Autodesk Inventor part; units mm, degrees
ref_plane "YZ Plane" through (0, 0, 0) normal (1, 0, 0) x (0, 1, 0)
ref_plane "XZ Plane" through (0, 0, 0) normal (0, 1, 0) x (-1, 0, 0)
ref_plane "XY Plane" through (0, 0, 0) normal (0, 0, 1) x (1, 0, 0)
sketch "Sketch1" plane through (0, 0, 0) normal (0, 1, 0) x (-1, 0, 0)
  line L0 (-31, -18.5) -> (31, -18.5)
  line L1 (31, -18.5) -> (31, 18.5)
  line L2 (31, 18.5) -> (-31, 18.5)
  line L3 (-31, 18.5) -> (-31, -18.5)
  line L4 (-31, -18.5) -> (31, 18.5) construction
  line L5 (31, -18.5) -> (-31, 18.5) construction
  line L6 (-35, -22) -> (35, -22)
  line L7 (35, -22) -> (35, 22)
  line L8 (35, 22) -> (-35, 22)
  line L9 (-35, 22) -> (-35, -22)
  line L10 (-35, -22) -> (35, 22) construction
  line L11 (35, -22) -> (-35, 22) construction
  line L12 (12.5, -32) -> (-12.5, -32)
  line L13 (0, -22) -> (12.5, -32) construction
  line L14 (0, -22) -> (-12.5, -32) construction
  line L15 (-12.5, 32) -> (12.5, 32)
  line L16 (12.5, 32) -> (12.5, 22)
  line L17 (-12.5, 22) -> (-12.5, 32)
  line L18 (-12.5, 32) -> (0, 22) construction
  line L19 (12.5, 32) -> (0, 22) construction
  line L20 (12.5, -22) -> (12.5, -32)
  line L21 (-12.5, -32) -> (-12.5, -22)
  line L22 (-12.5, -27) -> (12.5, -27)
  line L23 (-12.5, 27) -> (12.5, 27)
  line L24 (-35, -22) -> (-35, -18.5)
  line L25 (-35, 22) -> (-31, 22)
  line L26 (-35, 22) -> (-35, 18.5)
  point P0 (0, 0)
  dimension "d2" = 70
  dimension "d3" = 44
  dimension "d16" = 25
  dimension "d97" = 37
extrude "Extrusion2" add sketch "Sketch1" along normal blind 20 contours L9 L8 L7 L6
extrude "Extrusion3" add sketch "Sketch1" along normal blind 2 contours L3 L2 L1 L0
sketch "Sketch2" plane through (-35, 0, 22) normal (0, 0, 1) x (1, 0, 0)
  line L0 (66, 2) -> (66, 20)
  line L1 (4, 2) -> (4, 20)
  line L2 (66, 13.7796) -> (4, 13.7796)
  line L3 (4, 13.7796) -> (4, 6.7329)
  line L4 (4, 6.7329) -> (66, 6.7329)
  line L5 (66, 6.7329) -> (66, 13.7796)
  point P0 (35, 0)
extrude "Extrusion4" cut sketch "Sketch2" against normal blind 45
extrude "Extrusion5" add sketch "Sketch1" along normal blind 2 contours L6 L20 L22 L21 | L22 L20 L12 L21
extrude "Extrusion6" add sketch "Sketch1" along normal blind 2 contours L8 L17 L23 L16 | L23 L17 L15 L16
sketch "Sketch3" plane through (-12.5, 2, 32) normal (0, 0, 1) x (1, 0, 0)
  line L0 (2.5, -3.3793) -> (22.5, -3.3793)
  line L1 (22.5, -3.3793) -> (22.5, -4.9914)
  line L2 (22.5, -4.9914) -> (2.5, -4.9914)
  line L3 (2.5, -4.9914) -> (2.5, -3.3793)
  line L4 (25, -2) -> (25, 0)
  point P0 (12.5, -2)
  point P1 (25, -6)
  dimension "d28" = 20
  dimension "d29" = 2.5
extrude "Extrusion9" cut sketch "Sketch3" against normal blind 5
sketch "Sketch4" plane through (12.5, 2, -32) normal (0, 0, -1) x (-1, 0, 0)
  line L0 (2.5, -3.3796) -> (22.5, -3.3796)
  line L1 (22.5, -3.3796) -> (22.5, -4.9916)
  line L2 (22.5, -4.9916) -> (2.5, -4.9916)
  line L3 (2.5, -4.9916) -> (2.5, -3.3796)
  line L4 (25, -2) -> (25, 0)
  point P0 (12.5, -2)
  point P1 (25, -6)
  dimension "d32" = 20
  dimension "d34" = 2.5
extrude "Extrusion10" cut sketch "Sketch4" against normal blind 5
extrude "Extrusion11" add sketch "Sketch1" against normal blind 10 contours L9 L8 L7 L6
extrude "Extrusion12" add sketch "Sketch1" against normal blind 10 contours L3 L2 L1 L0
sketch "Sketch5" plane through (35, 20, 22) normal (1, 0, 0) x (0, 0, -1)
  line L0 (22, -20) -> (22, -110)
  circle A0 centre (22, -110) radius 90
  dimension "d42" = 90
  dimension "d43" = 180
extrude "Extrusion13" cut sketch "Sketch5" against normal blind 70
sketch "Sketch6" plane through (35, 20, -22) normal (0, 0, -1) x (-1, 0, 0)
  point P0 (35, -20)
sketch "Sketch7" plane through (0, 20, 0) normal (0, 1, 0) x (1, 0, 0)
  line L0 (-31, 18.5) -> (31, 18.5)
  line L1 (31, 18.5) -> (35, 18.5)
  line L2 (35, -22) -> (35, 22)
  line L3 (31, 18.5) -> (31, -18.5)
  line L4 (31, -18.5) -> (36, -18.5)
  point P0 (0, 0)
sketch "Sketch8" plane through (31, 20, -18.5) normal (-1, 0, 0) x (0, 0, 1)
  line L0 (0, 0) -> (0, -2)
  line L1 (0, -2) -> (37, -2)
  line L2 (37, -6.2204) -> (37, 0)
  line L3 (37, -2) -> (37, 0)
  line L4 (37, -5.0018) -> (37, -7.0018)
  line L5 (40.5, 0) -> (-3.5, 0)
  line L6 (37, -7.0018) -> (2, -7.0018)
  line L7 (2, -7.0018) -> (2, -5.0018)
  point P0 (18.5, -20)
  dimension "d46" = 2
  dimension "d47" = 2
sketch "Sketch14" plane through (0, 20, 0) normal (0, 1, 0) x (1, 0, 0)
  line L0 (31, 18.5) -> (31, 22)
  line L1 (31, 18.5) -> (35, 18.5)
  line L2 (35, -22) -> (35, 22)
  line L3 (31, 18.5) -> (31, -18.5)
  line L4 (31, -18.5) -> (35, -18.5)
  line L5 (35, -18.5) -> (35, 18.5)
  line L6 (31, 18.5) -> (31, -18.5)
  line L7 (-31, 18.5) -> (31, 18.5)
  line L8 (31, -18.5) -> (-31, -18.5)
  line L9 (31, -18.5) -> (31, -14.9394)
extrude "Extrusion18" cut sketch "Sketch14" against normal blind 2
sketch "Sketch21" plane through (35, -2.7303, -22) normal (0, 0, -1) x (-1, 0, 0)
  line L0 (66, 15.2303) -> (66, 19.6201)
  line L1 (66, 16.5099) -> (66, 22.7303)
  line L2 (66, 22.7303) -> (46, 22.7303)
  line L3 (46, 22.7303) -> (46, 15.2303)
  line L4 (46, 15.2303) -> (66, 15.2303)
  line L5 (66, 22.7303) -> (66, 15.2303)
  point P0 (35, 2.7303)
  dimension "d84" = 7.5
  dimension "d91" = 20
sketch "Sketch25" plane through (31, 6.7329, -22) normal (0, 0, -1) x (-1, 0, 0)
  line L0 (0, 7.0467) -> (62, 7.0467)
  line L1 (0, 7.0467) -> (0, 13.2671)
  line L2 (66, 13.2671) -> (-4, 13.2671)
  line L3 (0, 13.2671) -> (20, 13.2671)
  line L4 (20, 13.2671) -> (20, 5.7671)
  line L5 (20, 5.7671) -> (0, 5.7671)
  line L6 (0, 5.7671) -> (0, 13.2671)
  point P0 (31, -6.7329)
  dimension "d98" = 20
  dimension "d99" = 7.5
extrude "Extrusion29" add sketch "Sketch1" against normal blind 6 contours L22 L20 L12 L21
extrude "Extrusion30" add sketch "Sketch1" against normal blind 6 contours L23 L17 L15 L16
sketch "Sketch28" plane through (12.5, 2, -32) normal (0, 0, -1) x (-1, 0, 0)
  line L0 (2, -3.2303) -> (23, -3.2303)
  line L1 (23, -3.2303) -> (23, -6.2303)
  line L2 (23, -6.2303) -> (2, -6.2303)
  line L3 (2, -6.2303) -> (2, -3.2303)
  line L4 (-22.5, -4.7303) -> (47.5, -4.7303)
  line L5 (2, -3.2303) -> (23, -6.2303) construction
  line L6 (23, -3.2303) -> (2, -6.2303) construction
  point P0 (12.5, -2)
  point P1 (12.5, -4.7303)
  dimension "d111" = 21
  dimension "d112" = 3
extrude "Extrusion31" cut sketch "Sketch28" against normal blind 6
sketch "Sketch29" plane through (-12.5, 2, 32) normal (0, 0, 1) x (1, 0, 0)
  line L0 (2, -3.2303) -> (23, -3.2303)
  line L1 (2, -6.2303) -> (23, -6.2303)
  line L2 (23, -6.2303) -> (23, -3.2303)
  line L3 (23, -3.2303) -> (2, -3.2303)
  line L4 (2, -3.2303) -> (2, -6.2303)
  line L5 (47.5, -4.7303) -> (-22.5, -4.7303)
  line L6 (2, -6.2303) -> (23, -3.2303) construction
  line L7 (23, -6.2303) -> (2, -3.2303) construction
  point P0 (12.5, -2)
  point P1 (12.5, -4.7303)
  dimension "d115" = 21
extrude "Extrusion32" cut sketch "Sketch29" against normal blind 6
sketch "Sketch30" plane through (-12.5, 0, -22) normal (-1, 0, 0) x (0, 0, 1)
  point P0 (22, 0)
extrude "Extrusion33" cut sketch "Sketch1" along normal blind 6.75 contours L8 L17 L23 L16 | L23 L17 L15 L16
extrude "Extrusion34" add sketch "Sketch1" along normal blind 6.75 contours L23 L17 L15 L16
extrude "Extrusion35" add sketch "Sketch1" along normal blind 6.75 contours L8 L17 L23 L16
extrude "Extrusion36" cut sketch "Sketch1" along normal blind 6.75 contours L6 L20 L22 L21
extrude "Extrusion37" add sketch "Sketch1" along normal blind 6.75 contours L6 L20 L22 L21 | L22 L20 L12 L21
extrude "Extrusion38" add sketch "Sketch25" along normal blind 10
extrude "Extrusion39" add sketch "Sketch21" along normal blind 10
sketch "Sketch32" plane through (-31, 13.7796, -22) normal (-1, 0, 0) x (0, 0, 1)
  line L0 (-10, 6.2204) -> (-10, -1.2796)
  line L1 (-6, 2.4704) -> (0, 2.4704)
  line L2 (0, -16.5099) -> (0, 6.2204)
  line L3 (-6, 2.4704) -> (-6, -1.2796)
  line L4 (0, -1.2796) -> (-10, -1.2796)
  line L5 (-6, -1.2796) -> (0, -1.2796)
  line L6 (0, 2.4704) -> (0, -1.2796)
  point P0 (22, -13.7796)
extrude "Extrusion40" cut sketch "Sketch32" against normal blind 20
sketch "Sketch33" plane through (31, 13.7796, -22) normal (1, 0, 0) x (0, 0, -1)
  line L0 (10, -1.2796) -> (10, 6.2204)
  line L1 (0, 2.4704) -> (6, 2.4704)
  line L2 (6, 2.4704) -> (6, -1.2796)
  line L3 (6, 2.4704) -> (6, -1.2796)
  line L4 (6, -1.2796) -> (6, 2.4704)
  line L5 (6, -1.2796) -> (0, -1.2796)
  line L6 (0, -1.2796) -> (0, 2.4704)
  line L7 (6, 2.4704) -> (0, 2.4704)
  point P0 (-22, -13.7796)
extrude "Extrusion41" cut sketch "Sketch33" against normal blind 20
sketch "Sketch34" plane through (0, 20, 0) normal (0, 1, 0) x (1, 0, 0)
  point P0 (0, 0)
properties part number "kotelon alaosa"
Geometry: final body of the model. Coordinates: model frame, mm. A direction names the side the tool comes from. Coordinates: 2 decimals unless noted, no trailing zeros. Order: outer loops, then holes, each group sorted by start corner. A loop starts at its lowest first (then second) coordinate and runs counter-clockwise, first axis right, second up. Notation, with made-up numbers: (7, 89) - (50, 89) arc R14 cw to (50, 99) - close; hole circle Ø6 at (29.25, -6.75). An arc over 180 degrees is marked (long way). Return JSON: item names as keys, results as strings. Group by question number.
1. Cut plane B-B (y = 9). Output: boundary loops of the cut face in (x, z), plus the area to 3 significant figures.
2. Set-up query: faces 1 (the face through (-10.5, -3, -30)), 2 (the face through (31, 17, -28)), 3 (the face through (0, -5, -27)). Return all of +Z, -Z, +X, -X, +Y, -Y with unobstructed straight access to the full face (end or side cutting, diameter ignored); none if empty.
3. Cut plane D-D (z = 21). Output: boundary loops of the cut face in (x, y).
4. Material intervals for line 1 along Z through (x, y) = (-6, 6.5); line 2 along X through (y, z) = (13.25, -28.5); line 3 along X through (y, z) = (9, -5.5), sorted ascending. Write a range as [from, to].
5. Cut plane C-C (y = 5.25). Output: boundary loops of the cut face in (x, z), plus the area to 3 significant figures.
6. Pull-direction query (X, two-part tool) for faces 4 (the face through (12.5, 2, -28)), 5 (the face through (-12.5, 2, 28)), 6 (the face through (-21, 16.25, -25)), 7 (the face through (0, 6.733, 20)); classes: pulls with the +X half, pulls with the -X half, needs draft (parallel to the pull), parting line crosses it, or undercut.
7. Cut plane A-A (x = 19). Output: boundary loops of the cut face in (y, z), plus the area to 3 significant figures.
8. Pin query (flat end, axial travel): pin 1 (5 mm diameter, centred on x = 1.5, z = -3, fed in from -Y); pin 2 (2 mm diameter, centred on x = 33, z = 6.5, fed in from +Y); pin 3 (4 mm diameter, centred on y = 14.5, z = -27.5, fed in from -X). Return the tip coordinate at first contact, or that it passes through.
Resolved:
{
 "1": {"outline": "(-35, -22) - (-31, -22) - (-31, 22) - (-35, 22) - close; (31, -22) - (35, -22) - (35, 22) - (31, 22) - close", "area": "352 mm²"},
 "2": {"face 1": "-Z", "face 2": "-Z, +X, +Y, -Y", "face 3": "+X, -X, -Y"},
 "3": {"outline": "(-35, -2.48) - (35, -2.48) - (35, 20) - (-35, 20) - close; hole (-31, 6.73) - (31, 6.73) - (31, 13.78) - (-31, 13.78) - close"},
 "4": {"line 1": "z = [-32, -18.5], [18.5, 32]", "line 2": "x = [-31, -11], [11, 31]", "line 3": "x = [-35, -31], [31, 35]"},
 "5": {"outline": "(-35, -22) - (-12.5, -22) - (-12.5, -32) - (12.5, -32) - (12.5, -22) - (35, -22) - (35, 22) - (12.5, 22) - (12.5, 32) - (-12.5, 32) - (-12.5, 22) - (-35, 22) - close; hole (-31, -18.5) - (31, -18.5) - (31, 18.5) - (-31, 18.5) - close", "area": "1,290 mm²"},
 "6": {"face 4": "pulls with the +X half", "face 5": "pulls with the -X half", "face 6": "needs draft", "face 7": "undercut"},
 "7": {"outline": "(-2.73, -22) - (6.73, -22) - (6.73, -18.5) - (2, -18.5) - (2, 18.5) - (6.73, 18.5) - (6.73, 22) - (-2.73, 22) arc R90 cw to start; (12.5, -32) - (20, -32) - (20, -18.5) - (13.78, -18.5) - (13.78, -22) - (16.25, -22) - (16.25, -28) - (12.5, -28) - close; (13.78, 18.5) - (20, 18.5) - (20, 22) - (13.78, 22) - close", "area": "257 mm²"},
 "8": {"pin 1": "stops at y = -0.17", "pin 2": "stops at y = 18", "pin 3": "stops at x = -31"}
}
